Check sheet for the modelled part. Datum: model origin and axes. Units: mm. A direction names the side the tool comes from. Give positions to 0.01 mm unless a question says otherwise; leave off trailing zeros. Order: outer loops, then holes, each group sorted by start corner. A loop starts at its lowest first (then second) coordinate and runs counter-clockwise, first axis right, second up.
from build123d import *

# Parameters (mm, degrees)
F0_W     = 127
F0_H     = 177.8
F1_DEPTH = 1.5875
F2_DEPTH = 9.525
F3_DEPTH = 6.35
F4_D     = 3.175


with BuildPart() as f1:
    # F0 (on Front) → F1 (new body)
    with BuildSketch(Plane.XZ):
        with Locations((-37.948684603, 39.8532302618)):
            Rectangle(F0_W, F0_H)
        Polygon((-96.8245146513, 59.2209026217), (-96.8245146513, 122.7209026217), (-20.6245146513, 122.7209026217), (-20.6245146513, 59.2209026217), (-20.6245146513, 8.4209026217), (-96.8245146513, 8.4209026217), align=None, mode=Mode.SUBTRACT)
    extrude(amount=F1_DEPTH)

    # F0 (on Front) → F2 (join)
    with BuildSketch(Plane.XZ):
        Polygon((-20.6245146513, 122.7209026217), (-96.8245146513, 122.7209026217), (-96.8245146513, 59.2209026217), (-58.7245146513, 59.2209026217), (-20.6245146513, 59.2209026217), align=None)
    extrude(amount=F2_DEPTH)

    # F0 (on Front) → F3 (join)
    with BuildSketch(Plane.XZ):
        Polygon((-58.7245146513, 59.2209026217), (-96.8245146513, 59.2209026217), (-96.8245146513, 8.4209026217), (-20.6245146513, 8.4209026217), (-20.6245146513, 59.2209026217), align=None)
        Polygon((-85.7120146513, 43.1527666092), (-58.7245146513, 43.1527666092), (-31.7370146513, 43.1527666092), (-31.7370146513, 17.7527666092), (-85.7120146513, 17.7527666092), align=None, mode=Mode.SUBTRACT)
        Polygon((-31.7370146513, 43.1527666092), (-58.7245146513, 43.1527666092), (-85.7120146513, 43.1527666092), (-85.7120146513, 17.7527666092), (-31.7370146513, 17.7527666092), align=None)
    extrude(amount=F3_DEPTH)

    # F4 (through all)
    with Locations(Plane(origin=(0, 0, 0), x_dir=(1, 0, 0), z_dir=(0, 1, 0))):
        with Locations((-71.4245146513, -106.8459026217), (-44.4370146513, -106.8459026217), (-44.4370146513, -90.9709026217), (-71.4245146513, -90.9709026217), (-79.8828303814, -37.4092385173), (-79.8828303814, -24.7092385173)):
            Hole(F4_D / 2)


solid = f1.part
1) Section check A-A, the plane y = -4.5. Record the cut outline in (x, z) (1 decimal), then the cut area to 3 significant figures.
Recorded:
outline: (-96.8, 8.4) - (-20.6, 8.4) - (-20.6, 122.7) - (-96.8, 122.7) - close; hole circle Ø3.2 at (-79.9, 24.7); hole circle Ø3.2 at (-79.9, 37.4); hole circle Ø3.2 at (-71.4, 91); hole circle Ø3.2 at (-71.4, 106.8); hole circle Ø3.2 at (-44.4, 91); hole circle Ø3.2 at (-44.4, 106.8)
area: 8,660 mm2
2) Section check D-D, the plane z = 80. Record the cut outline in (x, y) (1 decimal).
Recorded:
outline: (-101.4, -1.6) - (-96.8, -1.6) - (-96.8, -9.5) - (-20.6, -9.5) - (-20.6, -1.6) - (25.6, -1.6) - (25.6, 0) - (-101.4, 0) - close
3) Material ranges on L1, parallel to Z at x = -90, y = -6; L2, parallel to Y at x = -2, z = -7.5; L3, parallel to X at y = -3.75, z = 71, recorded low to high.
Recorded:
L1: z = 8.42 to 122.72
L2: y = -1.59 to 0
L3: x = -96.82 to -20.62
4) Set-up check for faces 1 (the face through (-20.625, -5, 77)), 2 (the face through (-39, 0, 41)), 3 (the face through (-96.825, -5, 79)), 4 (the face through (-59, -6.35, 34)), 5 (the face through (-58, -6, 122.721)): record each of +Z, -Z, +X, -X, +Y, -Y from which the full face is reachable in a straight line by a thin tool's end or side.
Recorded:
face 1: +Z, -Z, +X, -Y
face 2: +Z, -Z, +X, -X, +Y
face 3: +Z, -Z, -X, -Y
face 4: -Z, +X, -X, -Y
face 5: +Z, +X, -X, -Y
5) Section check C-C, the plane z = 54. Record the cut outline in (x, y).
Recorded:
outline: (-101.45, -1.59) - (-96.82, -1.59) - (-96.82, -6.35) - (-20.62, -6.35) - (-20.62, -1.59) - (25.55, -1.59) - (25.55, 0) - (-101.45, 0) - close
6) Depth check by flat-ended pin: pin 1 Ø3 at (x, y) = (-33, -5.5) entering from -Z; pin 2 Ø3 at (y, z) = (-5.5, 99.5) entering from +X; pin 3 Ø12 at (x, z) = (-57.5, 60.5) entering from +Y; pin 4 Ø3 at (y, z) = (-7.5, 12.5) entering from -X. Enter the tip coordinate at first touch or a pass-through.
Recorded:
pin 1: stops at z = 8.42
pin 2: stops at x = -20.62
pin 3: stops at y = 0
pin 4: stops at x = -96.82
